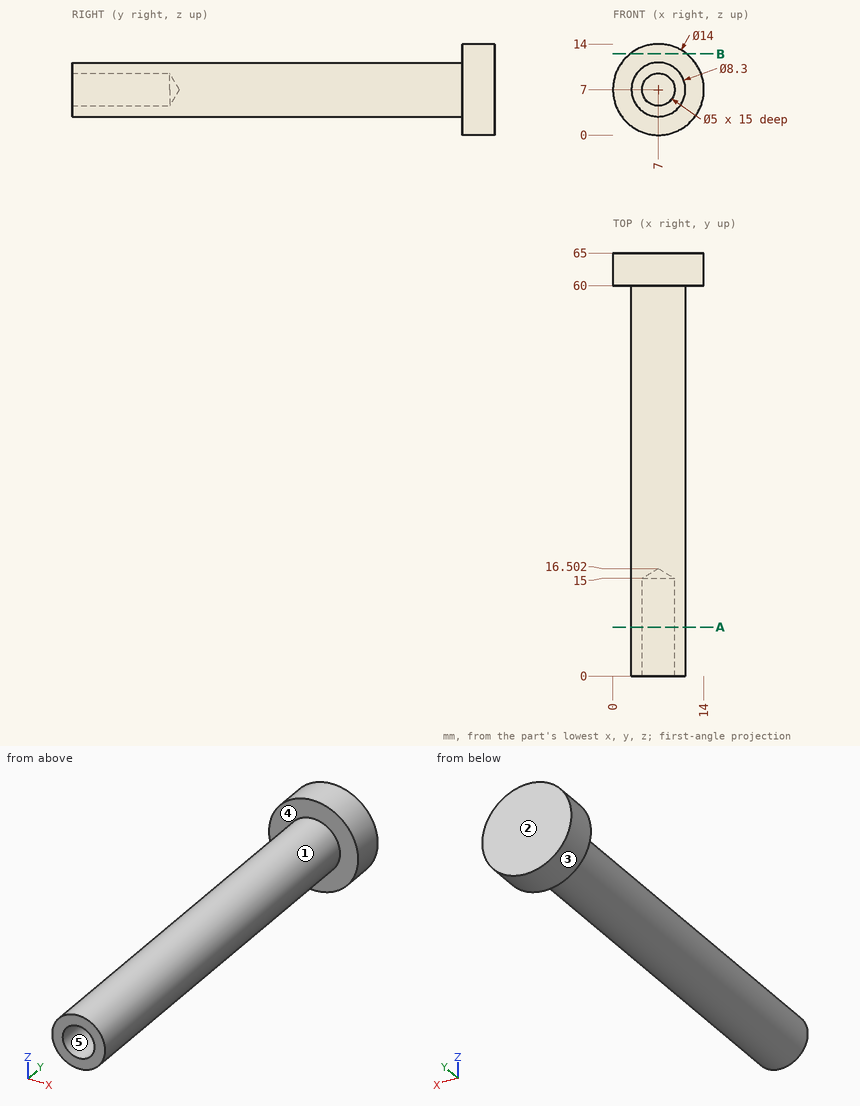
Design review of the part shown in the three views and the two pictorial views. Dimensions are in mm from the part's minimum x, y and z. A direction names the side the tool comes from. Give positions to 0.01 mm unless a question says otherwise; leave off trailing zeros. Write each loop counter-clockwise with the first axis right and the second up, starting at its lowest first coordinate (ties: lowest second). Pieces come first, ordered by that corner, then holes. Notation, with made-up numbers: M 54,-15.5 L 69,-15.5 A22 ccw 69,-3.5 Z; hole C 7.25,79.5 d6. An arc over 180 degrees is marked long. Answer as CSV lines item,"result".
1. Draft analysis for pull direction Z (two halves, no side actions). For the marked faces 3, 4 and 5, state which applies: +Z half, -Z half, draft (parallel to the pull), parting line (faces both ways), or undercut.
Findings:
face 3,"parting line"
face 4,"draft"
face 5,"undercut"
2. For the marked faces 1 and 2, list the 3-axis set-ups (+Z, -Z, +X, -X, +Y, -Y) from which the entire face can be reached by the end or side of a thin tool; tool diameter is ignored.
Findings:
face 1,"-Y"
face 2,"+Z, -Z, +X, -X, +Y"
3. Consider section A-A, the plane y = 7.5. Write out the cut boundary in (x, z).
Findings:
outline,"C 7,7 d8.3; hole C 7,7 d5"
4. Wall thickness on line 1 (Z direction, x = 7, y = 6.5); line 2 (Y direction, x = 4.5, z = 1.5); line 3 (X direction, y = 8.5, z = 6): over which ranges is each line inside the solid? List them lowest first.
Findings:
line 1,"z = 2.85 to 4.5, 9.5 to 11.15"
line 2,"y = 60 to 65"
line 3,"x = 2.97 to 4.71, 9.29 to 11.03"
5. Consider section B-B, the plane z = 12.5. Write out the cut boundary in (x, y), then the cut area to 3 significant figures.
Findings:
outline,"M 2.67,60 L 11.33,60 L 11.33,65 L 2.67,65 Z"
area,"43.3 mm2"
6. For pin 1 (1.5 mm diameter, centred on y = 26, z = 3.5, fed in from +X); pin 2 (6 mm diameter, centred on y = 27.5, z = 9.5, fed in from +X); pin 3 (4 mm diameter, centred on y = 44.5, z = 2.5, fed in from -X); pin 4 (2 mm diameter, centred on x = 6.5, z = 5.5, fed in from -Y), all flat-tipped, find the tip position at first contact; note any pin that passes through.
Findings:
pin 1,"stops at x = 10.11"
pin 2,"stops at x = 11.15"
pin 3,"stops at x = 3.69"
pin 4,"stops at y = 0"
